Geometry check sheet. Reference: the model listing, model coordinates, mm. A direction names the side the tool comes from. Coordinates: 2 decimals unless noted, no trailing zeros. Loops run counter-clockwise (first coordinate to the right, second up) from the corner with the lowest first, then second, coordinate; pieces in that order, holes last. Notation, with made-up numbers: (61.5, -30.75) - (83.5, -30.75) arc R27 cw to (83.5, 1.25) - close; hole circle Ø5 at (-25.75, 27). An arc over 180 degrees is marked (long way). Write each question's results on one line, items separated by ' | '. Start each with the question number.
(1) Go/stop test with flat-tipped pins: pin 1 Ø3.5 at (x, z) = (4, 2.5) entering from +Y; pin 2 Ø1 at (y, z) = (17, 0) entering from +X; pin 3 Ø5 at (y, z) = (19, -3) entering from -X. Record where each tip stops, or that it passes through.
(2) Material ranges on probe 1 along Y at (x, z) = (0.5, -1.5); probe 2 along X at (y, z) = (22, 9.75); probe 3 along X at (y, z) = (22, -2.5), recorded low to high.
(3) Mould release check, pull along Z, two halves, no side actions. Record for faces 1 (the face through (2, 23, 0)), 2 (the face through (0, 20, 10)): pulls with the +Z half, pulls with the -Z half, needs draft (parallel to the pull), parting line crosses it, or undercut.
(4) Access from +Z, -Z, +X, -X, +Y, -Y to the whole of each face (thin tool, end or side, straight path). Record for faces 3 (the face through (0, 23, 2)), 4 (the face through (3.087, 20.972, 6.181)).
(5) Sectioned sample at B-B (y = 24.25). Enter the section's corners in (x, z).
(6) Sectioned sample at A-A (z = 3). Enter the section's corners in (x, y), plus the area to 3 significant figures.
(7) Sectioned sample at C-C (z = -4). Enter the section's corners in (x, y).
(8) Sectioned sample at D-D (z = 7.75). Enter the section's corners in (x, y).
from build123d import *

# Parameters (mm, degrees)
BOX_W     = 10
BOX_H     = 10
BOX_DEPTH = 10


with BuildPart() as cube:
    # Box → Box (new body)
    with BuildSketch(Plane.XY):
        with Locations((5, 5)):
            Rectangle(BOX_W, BOX_H)
    extrude(amount=BOX_DEPTH)


with BuildPart() as cut:
    # Sphere → Sphere (revolve)
    with BuildSketch(Plane.XZ):
        with BuildLine():
            ThreePointArc((0, -5), (5, 0), (0, 5))
            Line((0, 5), (0, -5))
        make_face()
    revolve(axis=Axis((0, 0, 0), (0, 0, 1)))

    # Cut: cut Cube
    add(cube.part, mode=Mode.SUBTRACT)


with BuildPart() as cut_1:
    # Cut placement: moved
    add(cut.part.moved(Location((0, 20, 0))))


with BuildPart() as fusion:
    # Cone → Cone (revolve)
    with BuildSketch(Plane.XZ.offset(-20)):
        Polygon((0, 0), (2, 0), (4, 10), (0, 10), align=None)
    revolve(axis=Axis((0, 20, 0), (0, 0, 1)))

    # Fusion: union Cut
    add(cut_1.part)


solid = fusion.part
Outcome:
1) pin 1: stops at y = 21.18 | pin 2: stops at x = 4.33 | pin 3: stops at x = -4.96
2) probe 1: y = 15.26 to 24.74 | probe 2: x = -3.41 to 3.41 | probe 3: x = -3.84 to 3.84
3) face 1: undercut | face 2: pulls with the +Z half
4) face 3: +X, +Y | face 4: none
5) outline: (0, 0) - (0, 2.63) arc R2.63 ccw (long way) to (2.63, 0) - close
6) outline: (0, 22.6) - (0, 24) arc R4 ccw (long way) to (4, 20) - (2.6, 20) arc R2.6 ccw to start | area: 43.0 mm2
7) outline: circle Ø6 at (0, 20)
8) outline: circle Ø7.1 at (0, 20)
